Geometry: final body of the model. Coordinates: model frame, mm. Round coordinates to 2 decimals unless told otherwise and drop trailing zeros. Loops run counter-clockwise (first coordinate to the right, second up) from the corner with the lowest first, then second, coordinate; pieces in that order, holes last. Notation, with made-up numbers: M -39.75,-28 L -3.75,-28 A23 ccw -3.75,-3 Z; hole C 20,-33.5 d11. An arc over 180 degrees is marked long. Return JSON: item names as keys, results as strings.
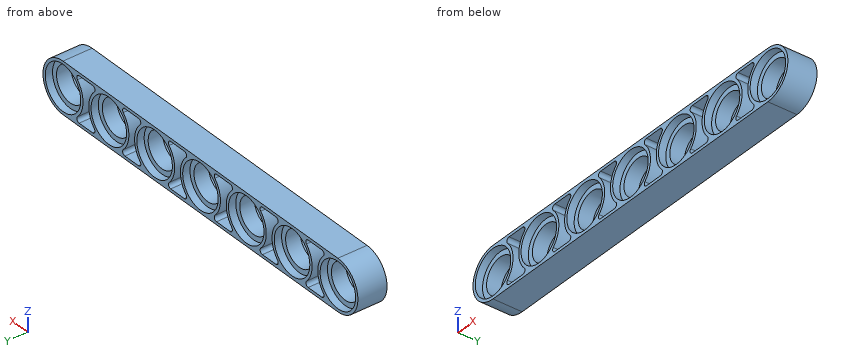
from build123d import *

# Parameters (mm, degrees)
BOSS_EXTRUDE1_DEPTH = 2
SKETCH2_R           = 3.1
CUT_EXTRUDE1_DEPTH  = 1
CUT_EXTRUDE2_START  = -1
SKETCH3_R           = 3.1
CUT_EXTRUDE2_DEPTH  = 1
SKETCH4_R           = 2.4
CUT_EXTRUDE3_DEPTH  = 52.705899083
LPATTERN1_COUNT     = 7
LPATTERN1_PITCH     = 8
CUT_EXTRUDE4_DEPTH  = 52.773545368
LPATTERN2_COUNT     = 6
LPATTERN2_PITCH     = 8


with BuildPart() as part:
    # Sketch1 → Boss-Extrude1 (new, symmetric)
    with BuildSketch(Plane(origin=(0, 0, 0), x_dir=(1, 0, 0), z_dir=(0, 1, 0))):
        with BuildLine():
            Line((0, 3.5), (48, 3.5))
            ThreePointArc((48, 3.5), (51.5, 0), (48, -3.5))
            Line((48, -3.5), (0, -3.5))
            ThreePointArc((0, -3.5), (-3.5, 0), (0, 3.5))
        make_face()
    extrude(amount=BOSS_EXTRUDE1_DEPTH, both=True)

    # Sketch2 → Cut-Extrude1 (cut)
    with BuildSketch(Plane(origin=(0, 2, 0), x_dir=(1, 0, 0), z_dir=(0, 1, 0))):
        with Locations(Location((0, 0, 0), (0, 0, 270))):
            Circle(SKETCH2_R)
    cut_extrude1 = extrude(amount=-CUT_EXTRUDE1_DEPTH, mode=Mode.SUBTRACT)

    # Sketch3 → Cut-Extrude2 (cut)
    with BuildSketch(Plane.XZ.offset(2).offset(CUT_EXTRUDE2_START)):
        with Locations(Location((0, 0, 0), (0, 0, 90))):
            Circle(SKETCH3_R)
    cut_extrude2 = extrude(amount=CUT_EXTRUDE2_DEPTH, mode=Mode.SUBTRACT)

    # Sketch4 → Cut-Extrude3 (cut, through all)
    with BuildSketch(Plane(origin=(0, 1, 0), x_dir=(1, 0, 0), z_dir=(0, 1, 0))):
        with Locations(Location((0, 0, 0), (0, 0, 270))):
            Circle(SKETCH4_R)
    cut_extrude3 = extrude(amount=-CUT_EXTRUDE3_DEPTH, mode=Mode.SUBTRACT)

    # LPattern1: Cut-Extrude1, Cut-Extrude2, Cut-Extrude3 ×7
    with Locations(*[(i * LPATTERN1_PITCH, 0, 0) for i in range(1, LPATTERN1_COUNT)]):
        add(cut_extrude1, mode=Mode.SUBTRACT)
        add(cut_extrude2, mode=Mode.SUBTRACT)
        add(cut_extrude3, mode=Mode.SUBTRACT)

    # Sketch5 → Cut-Extrude4 (cut, through all)
    with BuildSketch(Plane(origin=(0, 2, 0), x_dir=(1, 0, 0), z_dir=(0, 1, 0))):
        with BuildLine():
            Line((2.814249456, 3.1), (5.185750544, 3.1))
            ThreePointArc((5.185750544, 3.1), (5.553697029, 2.856892908), (5.474391514, 2.423076923))
            ThreePointArc((5.474391514, 2.423076923), (4.5, 0), (5.474391514, -2.423076923))
            ThreePointArc((5.474391514, -2.423076923), (5.553697029, -2.856892908), (5.185750544, -3.1))
            Line((5.185750544, -3.1), (2.814249456, -3.1))
            ThreePointArc((2.814249456, -3.1), (2.446302971, -2.856892908), (2.525608486, -2.423076923))
            ThreePointArc((2.525608486, -2.423076923), (3.5, 0), (2.525608486, 2.423076923))
            ThreePointArc((2.525608486, 2.423076923), (2.446302971, 2.856892908), (2.814249456, 3.1))
        make_face()
    cut_extrude4 = extrude(amount=-CUT_EXTRUDE4_DEPTH, mode=Mode.SUBTRACT)

    # LPattern2: Cut-Extrude4 ×6
    with Locations(*[(i * LPATTERN2_PITCH, 0, 0) for i in range(1, LPATTERN2_COUNT)]):
        add(cut_extrude4, mode=Mode.SUBTRACT)


solid = part.part
Q1. Section query A-A (x = 8). Output: boundary loops of the cut face in (y, z), plus the area to 3 significant figures.
Determined:
{"outline": "M -2,-3.5 L 2,-3.5 L 2,-3.1 L 1,-3.1 L 1,-2.4 L -1,-2.4 L -1,-3.1 L -2,-3.1 Z; M -2,3.1 L -1,3.1 L -1,2.4 L 1,2.4 L 1,3.1 L 2,3.1 L 2,3.5 L -2,3.5 Z", "area": "6.00 mm^2"}
Q2. Pin query (flat end, axial travel): pin 1 (1.5 mm diameter, centred on y = 0.5, z = -1.5, fed in from +X); pin 2 (1 mm diameter, centred on y = 1, z = -2.5, fed in from -X). Return the tip coordinate at first contact, or that it passes through.
Determined:
{"pin 1": "stops at x = 51.42", "pin 2": "stops at x = -2.87"}
Q3. Section query D-D (x = 23). Output: boundary loops of the cut face in (y, z).
Determined:
{"outline": "M -2,-3.5 L 2,-3.5 L 2,-2.93 L 1,-2.93 L 1,-2.18 L -1,-2.18 L -1,-2.93 L -2,-2.93 Z; M -2,2.93 L -1,2.93 L -1,2.18 L 1,2.18 L 1,2.93 L 2,2.93 L 2,3.5 L -2,3.5 Z"}
Q4. Material intervals for L1, parallel to Z at x = 21.5, y = 0.8; L2, parallel to Z at x = 3, y = 0.2; L3, parallel to Z at x = -1, y = -0.4, sorted ascending.
Determined:
{"L1": "z = -3.5 to -2.95, -2.45 to 2.45, 2.95 to 3.5", "L2": "z = -3.5 to -3.1, -1.8 to 1.8, 3.1 to 3.5", "L3": "z = -3.35 to -2.18, 2.18 to 3.35"}
Q5. Section query B-B (y = -0.1). State how many separate pieces and enclosed holes the cut face has, plus the area to 3 significant figures.
Determined:
{"separate pieces": "1", "enclosed holes": "13", "area": "176 mm^2"}
